Read the model definition and answer for the solid it produces. Units are mm, in the model's axes. A direction names the side the tool comes from. Give positions to 0.01 mm unless a question says otherwise; leave off trailing zeros. Order: outer loops, then holes, each group sorted by start corner. A loop starts at its lowest first (then second) coordinate and runs counter-clockwise, first axis right, second up. Notation, with made-up numbers: (-17, -32.5) - (14, -32.5) arc R21 cw to (14, -20.5) - close; hole circle Ø3 at (-30.75, 80). An arc over 180 degrees is marked (long way). Use a Markdown table: item, result. Add a question column.
1. A cutting plane is placed at D-D on y = -36. Determine the outline of the cut face in (x, z), and give its area (3 significant figures).
2. A cutting plane is placed at C-C on y = -8. Determine the outline of the cut face in (x, z), and give its area (3 significant figures).
3. A cutting plane is placed at B-B on y = 2. State how many separate pieces and enclosed holes the cut face has, and give its area (3 significant figures).
4. A cutting plane is placed at A-A on y = 23. Determine the outline of the cut face in (x, z).
5. Which of the six approach directions +Z, -Z, +X, -X, +Y, -Y give full straight-line access (tool end or side, diameter ignored) to faces 5 (the flat face through (11.4, -41, 12.2)), 6 (the cylindrical face through (7.501, -0.689, 9.307)), 7 (the cylindrical face through (18.04, -41.57, -1.4)), 8 (the cylindrical face through (-9.667, 25.451, -1.269))?
6. Consider L1, parallel to Z at x = -6, y = -1; L2, parallel to Z at x = 0, y = -25. Determine where each line is inside the solid, lowest interval first.
7. For a pull along X with two mould halves and no side action, classify faces 1 (the cylindrical face through (18, -48, 0)), 2 (the flat face through (11, 22, 0)), 3 (the flat face through (-2, -48, 18)), 4 (the flat face through (10, -1.2, 7.3)) as released by +X, released by -X, zero draft, split by the parting line, or undercut.
8. Flat-ended cylindrical pins translate along their axes: P1, Ø1, axis at y = 10, z = -12, coming from the -X side; P2, Ø4, axis at x = -9.5, y = 17, coming from the +Z side; P3, Ø1.1, axis at y = -48, z = 18.5, coming from the +X side. Find the tip coordinate at first contact, or state that the pin passes through.
```python
from build123d import *

# Parameters (mm, degrees)
BOSS_EXTRUDE1_DEPTH      = 29
BOSS_EXTRUDE1_DEPTH_BACK = 53
SKETCH2_R                = 20
CHAMFER1_SIZE            = 5
CHAMFER3_SIZE            = 1
CUT_EXTRUDE1_DEPTH       = 61.074953251
CUT_EXTRUDE1_DEPTH_BACK  = 61.074953251
CUT_EXTRUDE2_DEPTH       = 61.074953261
CUT_EXTRUDE2_DEPTH_BACK  = 61.074953261
SKETCH9_W                = 39.403997472
SKETCH9_H                = 4
CUT_EXTRUDE3_DEPTH       = 61.074953261
SKETCH10_W               = 32.489089837
SKETCH10_H               = 4
CUT_EXTRUDE5_DEPTH       = 61.074953261
SKETCH12_R               = 2.5
CUT_EXTRUDE6_DEPTH       = 27


with BuildPart() as part:
    # Sketch2 → Boss-Extrude1 (new, two sides: drawn at the far end of the back side and taken through both)
    with BuildSketch(Plane(origin=(0, 0, 0), x_dir=(1, 0, 0), z_dir=(0, 1, 0)).offset(-BOSS_EXTRUDE1_DEPTH_BACK)):
        with Locations(Location((0, 0, 0), (0, 0, 270))):
            Circle(SKETCH2_R)
    extrude(amount=BOSS_EXTRUDE1_DEPTH + BOSS_EXTRUDE1_DEPTH_BACK)

    # Chamfer1
    chamfer1_edges = [part.edges().sort_by_distance(p)[0] for p in [
        (0, 29, -20),
    ]]
    chamfer(chamfer1_edges, length=CHAMFER1_SIZE)

    # Sketch3 → Cut-Revolve1 (revolve, cut)
    with BuildSketch(Plane.XY, mode=Mode.PRIVATE) as cut_revolve1_sk:
        Polygon((20, 1.146940532), (20, 12.396940532), (10, 12.396940532), (10, 8.646940532), (-11, 8.646940532), (-15, 3.146940532), (-19, 3.146940532), (-19, 6.146940532), (-20, 6.146940532), (-20, 1.146940532), align=None)
    revolve(cut_revolve1_sk.sketch.rotate(Axis((-20, 1.146940532, 0), (1, 0, 0)), 180), axis=Axis((-20, 1.146940532, 0), (1, 0, 0)), mode=Mode.SUBTRACT)

    # Sketch4 → Cut-Revolve2 (revolve, cut)
    with BuildSketch(Plane(origin=(0, 0, 0), x_dir=(0, 0, -1), z_dir=(1, 0, 0))):
        Polygon((0, 13), (0, 29), (-9.75, 29), (-9.75, 22), (-16.25, 22), (-16.25, 13), align=None)
        Polygon((0, -53), (0, 1.146940532), (-7.5, 1.146940532), (-7.5, -12.6), (-9.75, -12.6), (-9.75, -14), (-16.25, -14), (-16.25, -53), align=None)
    revolve(axis=Axis((0, 29, 0), (0, -1, 0)), mode=Mode.SUBTRACT)

    # Chamfer3
    chamfer3_edges = [part.edges().sort_by_distance(p)[0] for p in [
        (0, -12.6, -7.5),
        (0, -12.6, -9.75),
        (0, -53, -16.25),
        (0, -53, -20),
    ]]
    chamfer(chamfer3_edges, length=CHAMFER3_SIZE)

    # Sketch5 → Cut-Extrude1 (cut, two sides: drawn at the far end of the back side and taken through both)
    with BuildSketch(Plane(origin=(0, 0, 0), x_dir=(0, 0, -1), z_dir=(1, 0, 0)).offset(-CUT_EXTRUDE1_DEPTH_BACK)):
        with BuildLine():
            Line((2, -43), (2, -46))
            ThreePointArc((2, -46), (0, -48), (-2, -46))
            Line((-2, -46), (-2, -43))
            ThreePointArc((-2, -43), (0, -41), (2, -43))
        make_face()
    extrude(amount=CUT_EXTRUDE1_DEPTH + CUT_EXTRUDE1_DEPTH_BACK, mode=Mode.SUBTRACT)

    # Sketch6 → Cut-Extrude2 (cut, two sides: drawn at the far end of the back side and taken through both)
    with BuildSketch(Plane.XY.offset(-CUT_EXTRUDE2_DEPTH_BACK)):
        with BuildLine():
            Line((2, -43), (2, -63))
            ThreePointArc((2, -63), (0, -65), (-2, -63))
            Line((-2, -63), (-2, -43))
            ThreePointArc((-2, -43), (0, -41), (2, -43))
        make_face()
    extrude(amount=CUT_EXTRUDE2_DEPTH + CUT_EXTRUDE2_DEPTH_BACK, mode=Mode.SUBTRACT)

    # Sketch9 → Cut-Extrude3 (cut, through all)
    with BuildSketch(Plane.XY):
        with Locations((19.701998736, -43)):
            Rectangle(SKETCH9_W, SKETCH9_H)
    extrude(amount=CUT_EXTRUDE3_DEPTH, mode=Mode.SUBTRACT)

    # Sketch10 → Cut-Extrude5 (cut, through all)
    with BuildSketch(Plane.XY):
        with Locations((-16.244544919, -43)):
            Rectangle(SKETCH10_W, SKETCH10_H)
    extrude(amount=-CUT_EXTRUDE5_DEPTH, mode=Mode.SUBTRACT)

    # Sketch12 → Cut-Extrude6 (cut)
    with BuildSketch(Plane.XZ.offset(14)):
        with Locations(Location((6.75, 11.691342951, 0), (0, 0, 270))):
            Circle(SKETCH12_R)
        with Locations(Location((-6.75, 11.691342951, 0), (0, 0, 270))):
            Circle(SKETCH12_R)
        with Locations(Location((6.75, -11.691342951, 0), (0, 0, 270))):
            Circle(SKETCH12_R)
        with Locations(Location((-6.75, -11.691342951, 0), (0, 0, 270))):
            Circle(SKETCH12_R)
    extrude(amount=-CUT_EXTRUDE6_DEPTH, mode=Mode.SUBTRACT)


solid = part.part
```
Output values:
| question | item | result |
|---|---|---|
| 1 | outline | circle Ø40 at (0, 0); hole circle Ø32.5 at (0, 0) |
| 1 | area | 427 mm² |
| 2 | outline | (10, -6.55) - (10, 6.55) - (18.9, 6.55) arc R20 ccw (long way) to (18.9, -6.55) - close; hole circle Ø5 at (-6.75, -11.69); hole circle Ø5 at (-6.75, 11.69); hole circle Ø15 at (0, 0); hole circle Ø5 at (6.75, -11.69); hole circle Ø5 at (6.75, 11.69) |
| 2 | area | 875 mm² |
| 3 | separate pieces | 2 |
| 3 | enclosed holes | 4 |
| 3 | area | 606 mm² |
| 4 | outline | circle Ø40 at (0, 0); hole circle Ø19.5 at (0, 0) |
| 5 | face 5 | +Z, +X |
| 5 | face 6 | -Y |
| 5 | face 7 | +Z, +X, -X |
| 5 | face 8 | +Y |
| 6 | L1 | -19.08 to -14.08, -9.31 to -7.19, 7.19 to 9.31, 14.08 to 19.08 |
| 6 | L2 | -20 to -16.25, 16.25 to 20 |
| 7 | face 1 | zero draft |
| 7 | face 2 | undercut |
| 7 | face 3 | undercut |
| 7 | face 4 | released by +X |
| 8 | P1 | x = -16.36 |
| 8 | P2 | z = 18.54 |
| 8 | P3 | x = 8.82 |
